Model file for the job. Use its own axes, mm. Face numbers are marked on the shaded views. A direction names the side the tool comes from. Give positions to 0.01 mm unless a question says otherwise; leave off trailing zeros. Write each loop counter-clockwise with the first axis right and the second up, starting at its lowest first coordinate (ties: lowest second). Pieces come first, ordered by that corner, then holes.
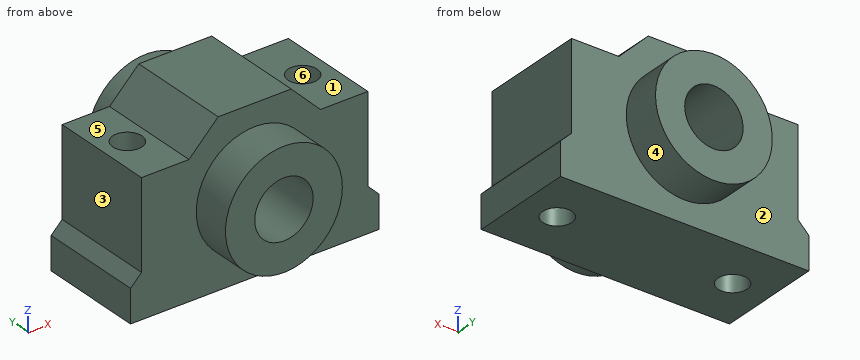
```python
from build123d import *

# Parameters (mm, degrees)
SKETCH_1_R               = 8
SKETCH_1_R_2             = 4
EXTRUDE_1_DEPTH          = 12.5
SKETCH_2_W               = 34
SKETCH_2_H               = 22
SKETCH_2_R               = 8
EXTRUDE_2_DEPTH          = 7.2
CUT_EXTRUDE_1_DEPTH      = 13.5
CUT_EXTRUDE_1_DEPTH_BACK = 13.5
SKETCH_4_OUTSIDE_W       = 45.518
SKETCH_4_OUTSIDE_H       = 36.518
SKETCH_4_OUTSIDE_R       = 2
CUT_EXTRUDE_2_DEPTH      = 1
CUT_EXTRUDE_2_DEPTH_BACK = 29.411764706


with BuildPart() as part:
    # 草图1 → 凸台-拉伸1 (new body, symmetric)
    with BuildSketch(Plane(origin=(0, 0, 0), x_dir=(1, 0, 0), z_dir=(0, 1, 0))):
        with Locations((-68.470588235, 17.411764706)):
            Circle(SKETCH_1_R)
        with Locations((-68.470588235, 17.411764706)):
            Circle(SKETCH_1_R_2, mode=Mode.SUBTRACT)
    extrude(amount=EXTRUDE_1_DEPTH, both=True)

    # 草图2 → 凸台-拉伸2 (add, symmetric)
    with BuildSketch(Plane(origin=(0, 0, 0), x_dir=(1, 0, 0), z_dir=(0, 1, 0))):
        with Locations((-68.470588235, 17.411764706)):
            Rectangle(SKETCH_2_W, SKETCH_2_H)
        with Locations((-68.470588235, 17.411764706)):
            Circle(SKETCH_2_R, mode=Mode.SUBTRACT)
    extrude(amount=EXTRUDE_2_DEPTH, both=True)

    # 草图3 → 切除-拉伸1 (cut, two sides)
    with BuildSketch(Plane(origin=(0, 0, 0), x_dir=(1, 0, 0), z_dir=(0, 1, 0))) as cut_extrude_1_sk:
        Polygon((-52.970588235, 22.411764706), (-52.970588235, 10.411764706), (-59.470588235, 10.411764706), (-63.470588235, 6.411764706), (-51.470588235, 6.411764706), (-51.470588235, 23.911764706), align=None)
        Polygon((-85.470588235, 6.411764706), (-73.470588235, 6.411764706), (-77.470588235, 10.411764706), (-83.970588235, 10.411764706), (-83.970588235, 22.411764706), (-85.470588235, 23.911764706), align=None)
    extrude(amount=CUT_EXTRUDE_1_DEPTH, mode=Mode.SUBTRACT)
    extrude(cut_extrude_1_sk.sketch, amount=-CUT_EXTRUDE_1_DEPTH_BACK, mode=Mode.SUBTRACT)

    # 草图4 outside → 切除-拉伸2 (cut, two sides)
    with BuildSketch(Plane.XY) as cut_extrude_2_sk:
        with Locations((-68.471, 0)):
            Rectangle(SKETCH_4_OUTSIDE_W, SKETCH_4_OUTSIDE_H)
        Polygon((-60.470588235, 7.2), (-60.470588235, 12.5), (-76.470588235, 12.5), (-76.470588235, 7.2), (-85.470588235, 7.2), (-85.470588235, -7.2), (-76.470588235, -7.2), (-76.470588235, -12.5), (-60.470588235, -12.5), (-60.470588235, -7.2), (-51.470588235, -7.2), (-51.470588235, 7.2), align=None, mode=Mode.SUBTRACT)
        with Locations((-56.470588235, 0)):
            Circle(SKETCH_4_OUTSIDE_R)
        with Locations((-80.470588235, 0)):
            Circle(SKETCH_4_OUTSIDE_R)
    extrude(amount=CUT_EXTRUDE_2_DEPTH, mode=Mode.SUBTRACT)
    extrude(cut_extrude_2_sk.sketch, amount=-CUT_EXTRUDE_2_DEPTH_BACK, mode=Mode.SUBTRACT)


solid = part.part
```
1. Pull direction X, two halves, no side cores. Call the marked faces 4, 5 and 6: +X half, -X half, draft (parallel to the pull), parting line (faces both ways), or undercut.
Calculated:
face 4: parting line
face 5: draft
face 6: undercut
2. Probe probe 1 along X at (y, z) = (7.75, -17.5); probe 2 along X at (y, z) = (1.75, -20); probe 3 along Y at (x, z) = (-54, -15). List the from-to ranges inside material, lowest first.
Calculated:
probe 1: x = -76.47 to -72.47, -64.47 to -60.47
probe 2: x = -83.97 to -81.44, -79.5 to -71.52, -65.42 to -57.44, -55.5 to -52.97
probe 3: y = -7.2 to 7.2
3. Pin check, flat tips, straight feed: P1, Ø1, axis at x = -76.5, y = -5.5, coming from the +Z side; P2, Ø1, axis at y = -5, z = -10, coming from the -X side; P3, Ø3, axis at y = -9, z = -23, coming from the +X side; P4, Ø6, axis at x = -64.5, z = -17.5, coming from the -Y side. Stop position of each tip, or through.
Calculated:
P1: stops at z = -8.94
P2: stops at x = -83.97
P3: stops at x = -61.59
P4: stops at y = -12.5
4. Slice it at C-C, the plane x = -54. Write the cut outline in (y, z).
Calculated:
outline: (-7.2, -28.41) - (7.2, -28.41) - (7.2, -10.41) - (-7.2, -10.41) - close
5. Slice it at D-D, the plane y = 9.5. Write the cut outline in (x, z), and give its area (3 significant figures).
Calculated:
outline: circle Ø16 at (-68.47, -17.41); hole circle Ø8 at (-68.47, -17.41)
area: 151 mm2
6. Slice it at B-B, the plane z = -20.5. Write the cut outline in (x, y).
Calculated:
outline: (-83.97, -7.2) - (-75.85, -7.2) - (-75.85, -12.5) - (-71.01, -12.5) - (-71.01, 12.5) - (-75.85, 12.5) - (-75.85, 7.2) - (-83.97, 7.2) - close; (-65.93, -12.5) - (-61.09, -12.5) - (-61.09, -7.2) - (-52.97, -7.2) - (-52.97, 7.2) - (-61.09, 7.2) - (-61.09, 12.5) - (-65.93, 12.5) - close; hole circle Ø4 at (-80.47, 0); hole circle Ø4 at (-56.47, 0)
7. Which spindle directions (+Z, -Z, +X, -X, +Y, -Y) get a long thin tool onto all of the face, cutting with end or side? Do the marked faces 1, 2 and 3. Say none if no direction does.
Calculated:
face 1: +Z, +X, +Y, -Y
face 2: +Y
face 3: +Z, -X, +Y, -Y
8. Slice it at A-A, the plane y = -1.5. Write the cut outline in (x, z), and give its area (3 significant figures).
Calculated:
outline: (-85.47, -28.41) - (-81.79, -28.41) - (-81.79, -10.41) - (-83.97, -10.41) - (-83.97, -22.41) - (-85.47, -23.91) - close; (-79.15, -28.41) - (-57.79, -28.41) - (-57.79, -10.41) - (-59.47, -10.41) - (-63.47, -6.41) - (-73.47, -6.41) - (-77.47, -10.41) - (-79.15, -10.41) - close; (-55.15, -28.41) - (-51.47, -28.41) - (-51.47, -23.91) - (-52.97, -22.41) - (-52.97, -10.41) - (-55.15, -10.41) - close; hole circle Ø8 at (-68.47, -17.41)
area: 484 mm2
